Work out the finished part from the listing and answer in its coordinate system (mm). A direction names the side the tool comes from. Coordinates: 2 decimals unless noted, no trailing zeros. Order: outer loops, then holes, each group sorted by start corner. A loop starts at its lowest first (then second) coordinate and runs counter-clockwise, first axis right, second up. Notation, with made-up numbers: M 57.25,27.5 L 80.25,27.5 A27 ccw 80.25,47.5 Z; hole C 84.25,9.25 d3. An arc over 180 degrees is marked long. Answer in a Markdown table with one row per item. Add a question column.
Item 1: The part is cut by section C-C (x = -17). Write down the section's boundary in (y, z), then the cut area to 3 significant figures.
Item 2: The part is cut by section D-D (y = -9.5). Write down the section's boundary in (x, z).
Item 3: Flat-ended cylindrical pins translate along their axes: pin 1 Ø7 at (x, z) = (70, 10) entering from -Y; pin 2 Ø10 at (y, z) = (23.5, 13.5) entering from -X; pin 3 Ø5 at (x, z) = (-50, 10) entering from -Y; pin 4 Ø6 at (y, z) = (-15, 10) entering from +X. Find the tip coordinate at first contact, or state that the pin passes through.
Item 4: Consider line 1 (Y direction, x = 65.5, z = 1); line 2 (Z direction, x = 58, y = -47); line 3 (Z direction, x = 70, y = 45). Determine where each line is inside the solid, lowest interval first. Write a range as from..to.
Item 5: The part is cut by section A-A (x = 46). Write down the section's boundary in (y, z).
Item 6: Which of the six approach directions +Z, -Z, +X, -X, +Y, -Y give full straight-line access (tool end or side, diameter ignored) to faces 4 (the face through (-45, -3.25, 10)), 5 (the face through (-15, 5, 10)), 6 (the face through (-45, 0, 13.25)), 7 (the face through (-15, 0, 5)), 8 (the face through (0, 1, 10))?
Item 7: The part is cut by section B-B (x = 70). Write down the section's boundary in (y, z), then the cut area to 3 significant figures.
Item 8: The mould has two halves that part along Z. Classify faces 1 (the face through (60.15, 44.57, 10.09)), 2 (the face through (-45, 0, 6.75)), 3 (the face through (45, -39.5, 10)): released by +Z, released by -Z, zero draft, split by the parting line, or undercut.
from build123d import *

# Parameters (mm, degrees)
EXTRUDE_1_DEPTH     = 20
SKETCH_3_W          = 10
SKETCH_3_H          = 10
SKETCH_3_W_2        = 6.5
SKETCH_3_H_2        = 6.5
EXTRUDE_2_DEPTH     = 10
EXTRUDE_START       = 10
SKETCH_3_3_W        = 6.5
SKETCH_3_3_H        = 6.5
EXTRUDE_3_DEPTH     = 50
SKETCH_4_W          = 20
SKETCH_4_H          = 10
EXTRUDE_4_DEPTH     = 12
SKETCH_2_R          = 2.15
SKETCH_2_R_2        = 2.75
CUT_EXTRUDE_1_DEPTH = 137.619910701


with BuildPart() as part:
    # 草图1 → 凸台-拉伸1 (new body)
    with BuildSketch(Plane.XY):
        Polygon((0, 39.5), (0, -39.5), (80, -39.5), (80, -49.5), (-10, -49.5), (-10, 49.5), (80, 49.5), (80, 39.5), align=None)
    extrude(amount=EXTRUDE_1_DEPTH)

    # 草图3 → 凸台-拉伸2 (add)
    # profile 1 of 2: a face of its own
    with BuildSketch(Plane.ZY.offset(10)):
        with Locations((10, 0)):
            Rectangle(SKETCH_3_W, SKETCH_3_H)
        with Locations((10, 0)):
            Rectangle(SKETCH_3_W_2, SKETCH_3_H_2, mode=Mode.SUBTRACT)
    # profile 2 of 2: a face of its own
    with BuildSketch(Plane.ZY.offset(10)):
        with Locations((10, 0)):
            Rectangle(SKETCH_3_W_2, SKETCH_3_H_2)
    extrude(amount=EXTRUDE_2_DEPTH)

    # 草图3<3> → 凸台-拉伸3 (add)
    with BuildSketch(Plane.ZY.offset(10).offset(EXTRUDE_START)):
        with Locations((10, 0)):
            Rectangle(SKETCH_3_3_W, SKETCH_3_3_H)
    extrude(amount=EXTRUDE_3_DEPTH)

    # 草图4 → 凸台-拉伸4 (add)
    with BuildSketch(Plane(origin=(80, 0, 0), x_dir=(0, 0, -1), z_dir=(1, 0, 0))):
        with Locations((-10, -44.5)):
            Rectangle(SKETCH_4_W, SKETCH_4_H)
        with Locations((-10, 44.5)):
            Rectangle(SKETCH_4_W, SKETCH_4_H)
    extrude(amount=EXTRUDE_4_DEPTH)

    # 草图2 → 切除-拉伸1 (cut, through all)
    with BuildSketch(Plane(origin=(0, 49.5, 0), x_dir=(1, 0, 0), z_dir=(0, 1, 0))):
        with Locations(Location((82, -10, 0), (0, 0, 180))):
            Circle(SKETCH_2_R)
        with BuildLine():
            Line((92, -20), (92, -10))
            ThreePointArc((92, -10), (89.071067812, -17.071067812), (82, -20))
            Line((82, -20), (92, -20))
        make_face()
        with BuildLine():
            ThreePointArc((82, 0), (89.071067812, -2.928932188), (92, -10))
            Line((92, -10), (92, 0))
            Line((92, 0), (82, 0))
        make_face()
        with Locations(Location((70, -10, 0), (0, 0, 180))):
            Circle(SKETCH_2_R_2)
        with Locations(Location((58, -10, 0), (0, 0, 180))):
            Circle(SKETCH_2_R)
    extrude(amount=-CUT_EXTRUDE_1_DEPTH, mode=Mode.SUBTRACT)


solid = part.part
Reply:
| question | item | result |
|---|---|---|
| 1 | outline | M -5,5 L 5,5 L 5,15 L -5,15 Z |
| 1 | area | 100 mm2 |
| 2 | outline | M -10,0 L 0,0 L 0,20 L -10,20 Z |
| 3 | pin 1 | stops at y = -49.5 |
| 3 | pin 2 | stops at x = -10 |
| 3 | pin 3 | stops at y = -3.25 |
| 3 | pin 4 | stops at x = 0 |
| 4 | line 1 | y = -49.5..-39.5, 39.5..49.5 |
| 4 | line 2 | z = 0..7.85, 12.15..20 |
| 4 | line 3 | z = 0..7.25, 12.75..20 |
| 5 | outline | M -49.5,0 L -39.5,0 L -39.5,20 L -49.5,20 Z; M 39.5,0 L 49.5,0 L 49.5,20 L 39.5,20 Z |
| 6 | face 4 | +Z, -Z, -X, -Y |
| 6 | face 5 | +Z, -Z, -X, +Y |
| 6 | face 6 | +Z, -X, +Y, -Y |
| 6 | face 7 | -Z, -X, +Y, -Y |
| 6 | face 8 | +Z, -Z, +X |
| 7 | outline | M -49.5,0 L -39.5,0 L -39.5,7.25 L -49.5,7.25 Z; M -49.5,12.75 L -39.5,12.75 L -39.5,20 L -49.5,20 Z; M 39.5,0 L 49.5,0 L 49.5,7.25 L 39.5,7.25 Z; M 39.5,12.75 L 49.5,12.75 L 49.5,20 L 39.5,20 Z |
| 7 | area | 290 mm2 |
| 8 | face 1 | undercut |
| 8 | face 2 | released by -Z |
| 8 | face 3 | zero draft |
